from build123d import *

# Parameters (mm, degrees)
IZIM1_R                          = 77.5
IZIM1_R_2                        = 60
IZIM1_R_3                        = 4.19
Y_KSEKLIK_EKSTR_ZYON1_DEPTH      = 10
IZIM2_R                          = 77.5
IZIM2_R_2                        = 60
Y_KSEKLIK_EKSTR_ZYON2_DEPTH      = 22
Y_KSEKLIK_EKSTR_ZYON3_START      = -10
IZIM3_R                          = 100
IZIM3_R_2                        = 60
Y_KSEKLIK_EKSTR_ZYON3_DEPTH      = 10
Y_KSEKLIK_EKSTR_ZYON4_REACH      = 210.384
Y_KSEKLIK_EKSTR_ZYON4_END_RADIUS = 77.5
IZIM5_W                          = 8.38
IZIM5_H                          = 22
DAIRESEL_KAPLAMA1_COUNT          = 4
EKSTR_ZYON_NCE4_DEPTH            = 4.19
DAIRESEL_KAPLAMA2_COUNT          = 4
IZIM7_R                          = 4.19
KES_EKSTR_ZYON1_DEPTH            = 10
IZIM8_R                          = 6
KES_EKSTR_ZYON2_DEPTH            = 144.122325303


with BuildPart() as part:
    # Çizim1 → Yükseklik-Ekstrüzyon1 (new body)
    with BuildSketch(Plane(origin=(0, 0, 0), x_dir=(1, 0, 0), z_dir=(0, 1, 0))):
        with Locations(Location((0, 0, 0), (0, 0, 270))):
            Circle(IZIM1_R)
        with Locations(Location((0, 0, 0), (0, 0, 270))):
            Circle(IZIM1_R_2, mode=Mode.SUBTRACT)
        with Locations(Location((0, 70, 0), (0, 0, 270))):
            Circle(IZIM1_R_3, mode=Mode.SUBTRACT)
        with Locations(Location((70, 0, 0), (0, 0, 270))):
            Circle(IZIM1_R_3, mode=Mode.SUBTRACT)
        with Locations(Location((0, -70, 0), (0, 0, 270))):
            Circle(IZIM1_R_3, mode=Mode.SUBTRACT)
        with Locations(Location((-70, 0, 0), (0, 0, 270))):
            Circle(IZIM1_R_3, mode=Mode.SUBTRACT)
    extrude(amount=Y_KSEKLIK_EKSTR_ZYON1_DEPTH)

    # Çizim2 → Yükseklik-Ekstrüzyon2 (add)
    with BuildSketch(Plane(origin=(0, 10, 0), x_dir=(1, 0, 0), z_dir=(0, 1, 0))):
        with Locations(Location((0, 0, 0), (0, 0, 270))):
            Circle(IZIM2_R)
        with Locations(Location((0, 0, 0), (0, 0, 270))):
            Circle(IZIM2_R_2, mode=Mode.SUBTRACT)
    extrude(amount=Y_KSEKLIK_EKSTR_ZYON2_DEPTH)

    # Çizim3 → Yükseklik-Ekstrüzyon3 (add)
    with BuildSketch(Plane(origin=(0, 32, 0), x_dir=(1, 0, 0), z_dir=(0, 1, 0)).offset(Y_KSEKLIK_EKSTR_ZYON3_START)):
        with Locations(Location((0, 0, 0), (0, 0, 270))):
            Circle(IZIM3_R)
        with Locations(Location((0, 0, 0), (0, 0, 270))):
            Circle(IZIM3_R_2, mode=Mode.SUBTRACT)
    extrude(amount=Y_KSEKLIK_EKSTR_ZYON3_DEPTH)

    # Yükseklik-Ekstrüzyon4: up to this cylinder (the profile starts outside it)
    y_kseklik_ekstr_zyon4_end = Plane(origin=(0, 11, 0), z_dir=(0, -1, 0)) * Cylinder(Y_KSEKLIK_EKSTR_ZYON4_END_RADIUS, 576.768, mode=Mode.PRIVATE)
    # Çizim5 → Yükseklik-Ekstrüzyon4 (add, up to the surface)
    with BuildSketch(Plane.XY.offset(80), mode=Mode.PRIVATE) as y_kseklik_ekstr_zyon4_sk1:
        with Locations((0, 11)):
            Rectangle(IZIM5_W, IZIM5_H)
    y_kseklik_ekstr_zyon4_tool1 = extrude(y_kseklik_ekstr_zyon4_sk1.sketch, amount=-Y_KSEKLIK_EKSTR_ZYON4_REACH, mode=Mode.PRIVATE) - y_kseklik_ekstr_zyon4_end
    y_kseklik_ekstr_zyon4 = y_kseklik_ekstr_zyon4_tool1.solids().sort_by_distance((0, 11, 80))[0]
    add(y_kseklik_ekstr_zyon4)

    # Dairesel Kaplama1: Yükseklik-Ekstrüzyon4 ×4 about axis
    dairesel_kaplama1_axis = Axis((0, 0, 0), (0, 1, 0))
    for i in range(1, DAIRESEL_KAPLAMA1_COUNT):
        add(y_kseklik_ekstr_zyon4.rotate(dairesel_kaplama1_axis, i * 360 / DAIRESEL_KAPLAMA1_COUNT))

    # Çizim6 → Ekstrüzyon-İnce4 (add, symmetric)
    with BuildSketch(Plane(origin=(0, 0, 0), x_dir=(0, 0, -1), z_dir=(1, 0, 0))):
        Polygon((-80, 0), (-90.601909395, 22), (-81.593384405, 26.341252988), (-70.99147501, 4.341252988), align=None)
    ekstr_zyon_nce4 = extrude(amount=EKSTR_ZYON_NCE4_DEPTH, both=True)

    # Dairesel Kaplama2: Ekstrüzyon-İnce4 ×4 about axis
    dairesel_kaplama2_axis = Axis((0, 0, 0), (0, 1, 0))
    for i in range(1, DAIRESEL_KAPLAMA2_COUNT):
        add(ekstr_zyon_nce4.rotate(dairesel_kaplama2_axis, i * 360 / DAIRESEL_KAPLAMA2_COUNT))

    # Çizim7 → Kes-Ekstrüzyon1 (cut)
    with BuildSketch(Plane.XZ):
        with Locations(Location((70, 0, 0), (0, 0, 90))):
            Circle(IZIM7_R)
        with Locations(Location((0, -70, 0), (0, 0, 90))):
            Circle(IZIM7_R)
        with Locations(Location((-70, 0, 0), (0, 0, 90))):
            Circle(IZIM7_R)
        with Locations(Location((0, 70, 0), (0, 0, 90))):
            Circle(IZIM7_R)
    extrude(amount=-KES_EKSTR_ZYON1_DEPTH, mode=Mode.SUBTRACT)

    # Çizim8 → Kes-Ekstrüzyon2 (cut, through all)
    with BuildSketch(Plane.XZ.offset(-22)):
        with Locations(Location((62.578950135, -62.578950135, 0), (0, 0, 270))):
            Circle(IZIM8_R)
        with Locations(Location((-62.578950135, -62.578950135, 0), (0, 0, 270))):
            Circle(IZIM8_R)
        with Locations(Location((-62.578950135, 62.578950135, 0), (0, 0, 270))):
            Circle(IZIM8_R)
        with Locations(Location((62.578950135, 62.578950135, 0), (0, 0, 270))):
            Circle(IZIM8_R)
    extrude(amount=-KES_EKSTR_ZYON2_DEPTH, mode=Mode.SUBTRACT)


solid = part.part
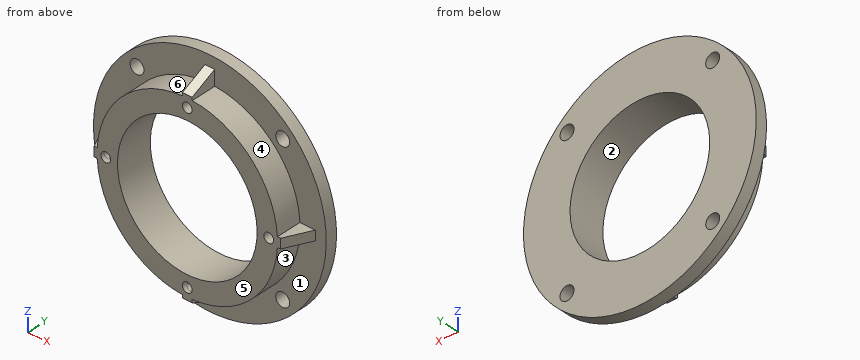
Source: CAD feature listing. Evaluate the final solid. Frame: model axes, mm. Face numbers are marked on the shaded views. A direction names the side the tool comes from. Round coordinates to 2 decimals unless told otherwise and drop trailing zeros. Loops run counter-clockwise (first coordinate to the right, second up) from the corner with the lowest first, then second, coordinate; pieces in that order, holes last. Notation, with made-up numbers: (42.25, 25) - (88.25, 25) arc R10 cw to (88.25, 42) - close; hole circle Ø3 at (59.25, 19.5). An arc over 180 degrees is marked (long way). Write item = value, one per line. Start each with the question number.
(1) Section query B-B, the plane y = 27.5. Output: boundary loops of the cut face in (x, z), plus the area to 3 significant figures.
(2) Set-up query: the marked faces 5 and 6. Return all of +Z, -Z, +X, -X, +Y, -Y with unobstructed straight access to the full face (end or side cutting, diameter ignored); none if empty.
(3) Pin query (flat end, axial travel): pin 1 (8 mm diameter, centred on y = 10, z = 11, fed in from -X); pin 2 (4 mm diameter, centred on x = -21, y = 11, fed in from +Z); pin 3 (15.5 mm diameter, centred on x = -62.58, z = -62.58, fed in from -Y). Return the tip coordinate at first contact, or that it passes through.
(4) Pull-direction query (Z, two-part tool) for the marked faces 1, 2, 3 and 4; classes: +Z half, -Z half, draft (parallel to the pull), parting line (faces both ways), or undercut.
(5) Section query A-A, the plane x = -25. Output: boundary loops of the cut face in (y, z).
(6) Ray query, line 1 along Y through (x, z) = (90, -31); line 2 along Z through (x, y) = (51.5, 30); line 3 along X through (y, z) = (4.25, 0). Return the intervals inside material, ascending. Write a range as from..to.
(7) Section query C-C, the plane x = 36.5. Output: boundary loops of the cut face in (y, z), plus the area to 3 significant figures.
Conclusion:
q1.outline = circle Ø200 at (0, 0); hole circle Ø12 at (-62.58, -62.58); hole circle Ø12 at (-62.58, 62.58); hole circle Ø120 at (0, 0); hole circle Ø12 at (62.58, -62.58); hole circle Ø12 at (62.58, 62.58)
q1.area = 19,700 mm2
q2.face_5 = +Z, -Z, +X, -X, -Y
q2.face_6 = +Z, -X, -Y
q3.pin_1 = -77.18
q3.pin_2 = 75.13
q3.pin_3 = 22
q4.face_1 = draft
q4.face_2 = undercut
q4.face_3 = -Z half
q4.face_4 = +Z half
q5.outline = (0, -73.36) - (22, -73.36) - (22, -96.82) - (32, -96.82) - (32, -54.54) - (0, -54.54) - close; (0, 54.54) - (32, 54.54) - (32, 96.82) - (22, 96.82) - (22, 73.36) - (0, 73.36) - close
q6.line_1 = 22..32
q6.line_2 = -85.72..-30.79, 30.79..85.72
q6.line_3 = -82.05..-74.19, -65.81..-60, 60..65.81, 74.19..82.05
q7.outline = (0, -68.37) - (22, -68.37) - (22, -93.1) - (32, -93.1) - (32, -47.62) - (0, -47.62) - close; (0, 47.62) - (32, 47.62) - (32, 93.1) - (22, 93.1) - (22, 68.37) - (0, 68.37) - close
q7.area = 1,820 mm2
